Geometry: see drawing. Coordinates: mm, zero at the bounding-box minimum. A direction names the side the tool comes from. Give positions to 0.01 mm unless a question says otherwise; leave off trailing zeros. Write each loop counter-clockwise with the first axis right and the second up, starting at its lowest first coordinate (ties: lowest second). Pieces come first, ordered by that corner, then holes. Notation, with made-up numbers: M -3.75,48 L 2.25,48 A31 ccw 2.25,74 Z; hole C 26,72 d6. An arc over 180 degrees is marked long. Use CSV: the item, a comma, the result in double quotes. Start each with the question number.
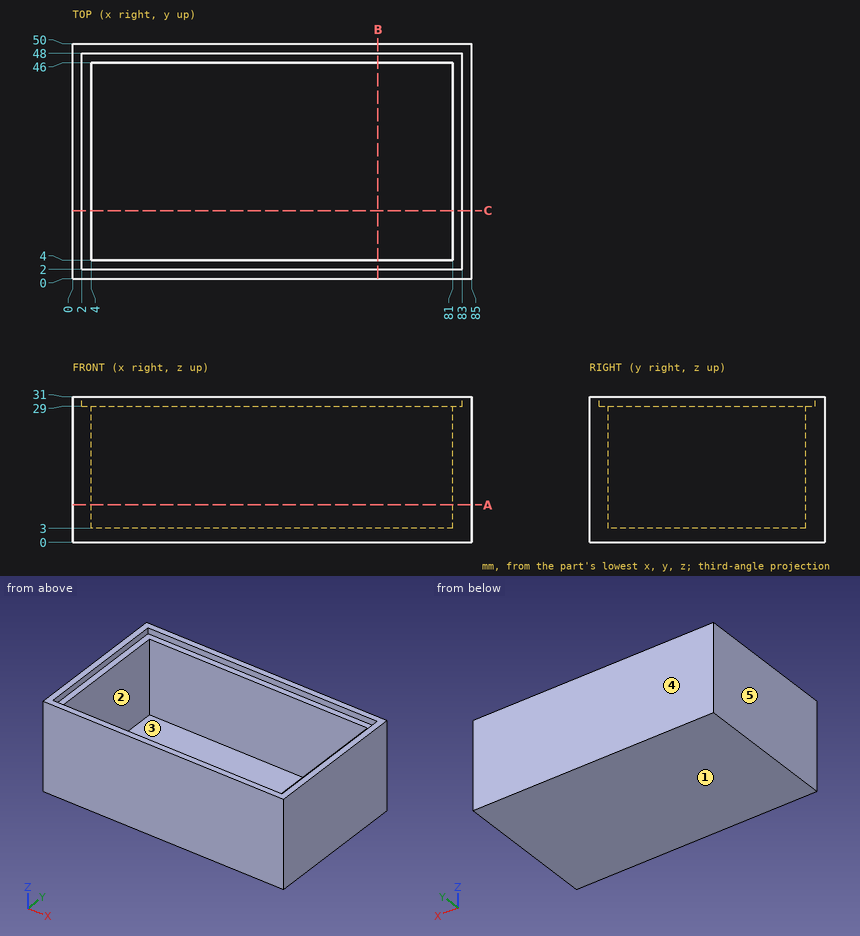
1. Section C-C on y = 14.5. Return loops of the section in (x, z).
2. Pull-direction query (Y, two-part tool) for the marked faces 3, 4 and 5; classes: released by +Y, released by -Y, zero draft, split by the parting line, or undercut.
3. Section A-A on z = 8. Return loops of the section in (x, y), then the cut area to 3 significant figures.
4. Section B-B on x = 65. Return loops of the section in (y, z).
5. Access query for the marked faces 1 and 2. Directions: +Z, -Z, +X, -X, +Y, -Y. A direction counts if a zero-diameter tool reaches every point of the face in a straight line with its end or side. Return the directions, or none.
6. Line query: probe 1 along X at (y, z) = (12, 18); probe 2 along Y at (x, z) = (30.5, 20); probe 3 along Z at (x, y) = (34, 31). Output: solid intervals per line, ascending.
Resolved:
1,outline,"M 0,0 L 85,0 L 85,31 L 83,31 L 83,29 L 81,29 L 81,3 L 4,3 L 4,29 L 2,29 L 2,31 L 0,31 Z"
2,face 3,"undercut"
2,face 4,"released by +Y"
2,face 5,"zero draft"
3,outline,"M 0,0 L 85,0 L 85,50 L 0,50 Z; hole M 4,4 L 81,4 L 81,46 L 4,46 Z"
3,area,"1,020 mm2"
4,outline,"M 0,0 L 50,0 L 50,31 L 48,31 L 48,29 L 46,29 L 46,3 L 4,3 L 4,29 L 2,29 L 2,31 L 0,31 Z"
5,face 1,"-Z, +X, -X, +Y, -Y"
5,face 2,"+Z"
6,probe 1,"x = 0 to 4, 81 to 85"
6,probe 2,"y = 0 to 4, 46 to 50"
6,probe 3,"z = 0 to 3"
